Model file for the job. Use its own axes, mm. Face numbers are marked on the shaded views. A direction names the side the tool comes from. Round coordinates to 2 decimals unless told otherwise and drop trailing zeros. Loops run counter-clockwise (first coordinate to the right, second up) from the corner with the lowest first, then second, coordinate; pieces in that order, holes last. Notation, with made-up numbers: M -22.75,-13.75 L 1.25,-13.75 A19 cw 1.25,22.25 Z; hole C 15,79 d2. An arc over 180 degrees is marked long. Answer in a Markdown table with one row per item.
from build123d import *

# Parameters (mm, degrees)
SKETCH_W     = 24
SKETCH_H     = 32
PAD_DEPTH    = 4
FILLET_R     = 4
SKETCH001_R  = 2.5
HOLE_DEPTH   = 25
SKETCH002_W  = 14
SKETCH002_H  = 6
POCKET_DEPTH = 5.2
PAD001_DEPTH = 6
FILLET001_R  = 1
FILLET002_R  = 1


with BuildPart() as part:
    # Sketch → Pad (new body, symmetric)
    with BuildSketch(Plane.XY):
        Rectangle(SKETCH_W, SKETCH_H)
    extrude(amount=PAD_DEPTH, both=True)

    # Fillet
    fillet_edges = [part.edges().sort_by_distance(p)[0] for p in [
        (-12, -16, 0),
        (12, -16, 0),
        (12, 16, 0),
        (-12, 16, 0),
    ]]
    fillet(fillet_edges, radius=FILLET_R)

    # Sketch001 (on Face5 of Fillet) → Hole (cut)
    with BuildSketch(Plane.XY.offset(4)):
        with Locations((-8, -4)):
            Circle(SKETCH001_R)
    hole = extrude(amount=-HOLE_DEPTH, mode=Mode.SUBTRACT)

    # Mirrored: Hole across Sketch001 V_Axis
    add(hole.mirror(Plane(origin=(0, 0, 4), x_dir=(0, 0, 1), z_dir=(1, 0, 0))), mode=Mode.SUBTRACT)

    # Sketch002 (on Face5 of Mirrored) → Pocket (cut)
    with BuildSketch(Plane.XY.offset(4)):
        with Locations((0, 13)):
            Rectangle(SKETCH002_W, SKETCH002_H)
    extrude(amount=-POCKET_DEPTH, mode=Mode.SUBTRACT)

    # Sketch003 (on Face16 of Pocket) → Pad001 (join)
    with BuildSketch(Plane.XY.offset(-1.2)):
        Polygon((7, 10), (-7, 10), (-7, 19.5), (-3, 19.5), (-3, 12), (3, 12), (3, 19.5), (7, 19.5), align=None)
    extrude(amount=PAD001_DEPTH)

    # Fillet001
    fillet001_edges = [part.edges().sort_by_distance(p)[0] for p in [
        (0, -16, -4),
        (10.828427, -14.828427, -4),
        (12, 0, -4),
        (10.828427, 14.828427, -4),
        (-10.828427, -14.828427, -4),
        (-12, 0, -4),
        (-10.828427, 14.828427, -4),
        (0, 16, -4),
    ]]
    fillet(fillet001_edges, radius=FILLET001_R)

    # Fillet002
    fillet002_edges = [part.edges().sort_by_distance(p)[0] for p in [
        (-10.828427, -14.828427, 4),
        (-12, 0, 4),
        (-10.828427, 14.828427, 4),
        (10.828427, 14.828427, 4),
        (12, 0, 4),
        (10.828427, -14.828427, 4),
        (0, -16, 4),
        (-7.5, 16, 4),
        (7.5, 16, 4),
    ]]
    fillet(fillet002_edges, radius=FILLET002_R)


solid = part.part
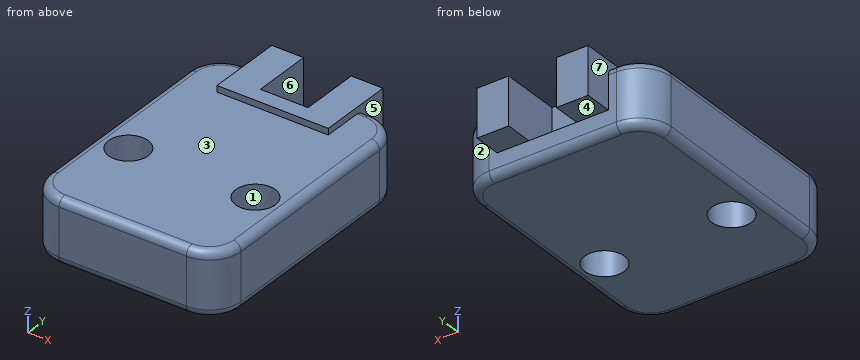
1. Mould opens along X. For the marked faces 1, 2 and 3 say: +X half, -X half, draft (parallel to the pull), parting line (faces both ways), or undercut.
Verdict:
| item | result |
|---|---|
| face 1 | undercut |
| face 2 | +X half |
| face 3 | draft |
2. Wall check: probe 1 along Y at (x, z) = (8, -1.5); probe 2 along X at (y, z) = (-2, 0); probe 3 along X at (y, z) = (-5.5, 3). Give the ranges that are in metal, low to high.
Verdict:
| item | result |
|---|---|
| probe 1 | y = -16 to -6.5, -1.5 to 16 |
| probe 2 | x = -12 to -9.5, -6.5 to 6.5, 9.5 to 12 |
| probe 3 | x = -12 to -10, -6 to 6, 10 to 12 |
3. Saw through at B-B (z = -2.25). Write the cut outline in (x, y), and give its area (3 significant figures).
Verdict:
| item | result |
|---|---|
| outline | M -12,-12 A4 ccw -8,-16 L 8,-16 A4 ccw 12,-12 L 12,12 A4 ccw 8,16 L -8,16 A4 ccw -12,12 Z; hole C -8,-4 d5; hole C 8,-4 d5 |
| area | 715 mm² |
4. Pin check, flat tips, straight feed: pin 1 (1.2 mm diameter, centred on x = -1, y = 13, fed in from +Z); pin 2 (1 mm diameter, centred on x = 4.5, y = 18, fed in from -Z); pin 3 (1.8 mm diameter, centred on y = 17.5, z = 0.5, fed in from +X); pin 4 (10 mm diameter, centred on x = -8.5, y = 10.5, fed in from +Z). Stop position of each tip, or through.
Verdict:
| item | result |
|---|---|
| pin 1 | stops at z = -1.2 |
| pin 2 | stops at z = -1.2 |
| pin 3 | stops at x = 7 |
| pin 4 | stops at z = 4.8 |
5. Saw through at A-A (y = -4). Write the cut outline in (x, z).
Verdict:
| item | result |
|---|---|
| outline | M -12,-3 A1 ccw -11,-4 L -10.5,-4 L -10.5,4 L -11,4 A1 ccw -12,3 Z; M -5.5,-4 L 5.5,-4 L 5.5,4 L -5.5,4 Z; M 10.5,-4 L 11,-4 A1 ccw 12,-3 L 12,3 A1 ccw 11,4 L 10.5,4 Z |
6. Tool access for the marked faces 4, 5, 6 and 7: list every direction of +Z, -Z, +X, -X, +Y, -Y with a clear straight run to the whole face (end or side of a thin tool).
Verdict:
| item | result |
|---|---|
| face 4 | -Z, +X, -X, +Y |
| face 5 | +Z, +X, +Y |
| face 6 | +Z, +Y |
| face 7 | +Z, -X, +Y |
7. Saw through at C-C (y = 10.5). Write the cut outline in (x, z).
Verdict:
| item | result |
|---|---|
| outline | M -12,-3 A1 ccw -11,-4 L 11,-4 A1 ccw 12,-3 L 12,3 A1 ccw 11,4 L 7,4 L 7,4.8 L -7,4.8 L -7,4 L -11,4 A1 ccw -12,3 Z |
